from build123d import *

# Parameters (mm, degrees)
F1_DEPTH = 12.7
F2_R     = 1.7272
F3_DEPTH = 12.7
F4_W     = 12.7
F4_H     = 28.575
F5_DEPTH = 6.35
F6_R     = 1.5875
F7_DEPTH = 6.35
F8_R     = 2.15265
F9_DEPTH = 12.7


with BuildPart() as f1:
    # F0 (on Top) → F1 (new body)
    with BuildSketch(Plane.XY):
        with BuildLine():
            Line((0, -508), (0, 0))
            ThreePointArc((0, 0), (-27.5469109355, 69.5607648032), (-95.25, 101.401368334))
            Line((-95.25, 101.401368334), (-95.25, 101.6))
            Line((-95.25, 101.6), (-107.95, 101.6))
            Line((-107.95, 101.6), (-107.95, 101.401368334))
            ThreePointArc((-107.95, 101.401368334), (-175.6530890645, 69.5607648032), (-203.2, 0))
            Line((-203.2, 0), (-203.2, -508))
            ThreePointArc((-203.2, -508), (-175.6530890645, -577.5607648032), (-107.95, -609.401368334))
            Line((-107.95, -609.401368334), (-107.95, -609.6))
            Line((-107.95, -609.6), (-95.25, -609.6))
            Line((-95.25, -609.6), (-95.25, -609.401368334))
            ThreePointArc((-95.25, -609.401368334), (-27.5469109355, -577.5607648032), (0, -508))
        make_face()
    extrude(amount=F1_DEPTH)

    # F2 (on face) → F3 (cut, through all)
    with BuildSketch(Plane.XY.offset(12.7)):
        with Locations((-32.54375, 63.404136047)):
            Circle(F2_R)
        with Locations((-32.54375, 42.766636047)):
            Circle(F2_R)
        with Locations((-170.65625, 42.766636047)):
            Circle(F2_R)
        with Locations((-170.65625, 63.404136047)):
            Circle(F2_R)
    extrude(amount=-F3_DEPTH, mode=Mode.SUBTRACT)

    # F4 (on face) → F5 (cut)
    with BuildSketch(Plane.XY.offset(12.7)):
        with Locations((-101.6, 87.3125)):
            Rectangle(F4_W, F4_H)
        with Locations((-101.6, -595.3125)):
            Rectangle(F4_W, F4_H)
    extrude(amount=-F5_DEPTH, mode=Mode.SUBTRACT)

    # F6 (on face) → F7 (cut, through all)
    with BuildSketch(Plane.XY.offset(12.7)):
        with Locations((-107.95, -581.025)):
            Circle(F6_R)
        with Locations((-95.25, -581.025)):
            Circle(F6_R)
        with Locations((-107.95, 73.025)):
            Circle(F6_R)
        with Locations((-95.25, 73.025)):
            Circle(F6_R)
    extrude(amount=-F7_DEPTH, mode=Mode.SUBTRACT)

    # F8 (on face) → F9 (cut, through all)
    with BuildSketch(Plane(origin=(0, 0, 0), x_dir=(1, 0, 0), z_dir=(0, 0, -1))):
        with Locations((-101.6, -96.8375)):
            Circle(F8_R)
        with Locations((-101.6, -77.7875)):
            Circle(F8_R)
        with Locations((-101.6, 604.8375)):
            Circle(F8_R)
        with Locations((-101.6, 585.7875)):
            Circle(F8_R)
    extrude(amount=-F9_DEPTH, mode=Mode.SUBTRACT)


solid = f1.part
Could you check a few things on this model? Use its own coordinates, in mm. Give positions to 0.01 mm unless a question says otherwise; leave off trailing zeros. Loops run counter-clockwise (first coordinate to the right, second up) from the corner with the lowest first, then second, coordinate; pieces in that order, holes last. Notation, with made-up numbers: (-34.75, 15) -> (7.25, 15) arc R11 cw to (7.25, 19) -> close; hole circle Ø11 at (79.25, 44.25). An arc over 180 degrees is marked (long way). Return JSON: item names as keys, results as strings.
Item 1: I'm going to push flat-ended pins straight in: pin 1 (7 mm diameter, centred on y = 83.5, z = 8, fed in from +X); pin 2 (2.5 mm diameter, centred on x = -107.95, y = -581.025, fed in from +Z); pin 3 (1 mm diameter, centred on x = -26, z = 9.5, fed in from -Y). Where does each tip first touch, or does it pass through?
Geometry results:
{"pin 1": "stops at x = -38.97", "pin 2": "stops at z = 6.35", "pin 3": "stops at y = -576.43"}
Item 2: If we section it at C-C on x = -54.5: List the corners of the cut face in (y, z) for me.
Geometry results:
{"outline": "(-598.02, 0) -> (90.02, 0) -> (90.02, 12.7) -> (-598.02, 12.7) -> close"}
Item 3: If we section it at A-A on z = 2: Count the separate pieces of the cut face and the enclosed holes in it, plus the area to 3 significant figures.
Geometry results:
{"separate pieces": "1", "enclosed holes": "8", "area": "136,000 mm²"}
Item 4: We'd pull the mould along X, two halves only. Please class faces 1 (the flat face through (-102, 87, 6.35)), 2 (the flat face through (-103, -249, 12.7)), 3 (the cylindrical face through (-28.285, -578.339, 6.261)): +X half, -X half, draft (parallel to the pull), parting line (faces both ways), or undercut.
Geometry results:
{"face 1": "undercut", "face 2": "draft", "face 3": "+X half"}
Item 5: If we section it at B-B on x = -141: List the corners of the cut face in (y, z) for me.
Geometry results:
{"outline": "(-601.65, 0) -> (93.65, 0) -> (93.65, 12.7) -> (-601.65, 12.7) -> close"}
Item 6: I need wall thicknesses on L1, parallel to Y at x = -101.6, z = 2.75; L2, parallel to Y at x = -31, z = 8.5; L3, parallel to X at y = -511.5, z = 10.25. Which ranges of each line are inside material? Lowest first, please. Write a range as from..to.
Geometry results:
{"L1": "y = -609.6..-606.99, -602.68..-587.94, -583.63..75.63, 79.94..94.68, 98.99..101.6", "L2": "y = -581.06..41.99, 43.54..62.63, 64.18..73.06", "L3": "x = -203.14..-0.06"}
